Autodesk Inventor part; units mm, degrees
ref_plane "YZ Plane" through (0, 0, 0) normal (1, 0, 0) x (0, 1, 0)
ref_plane "XZ Plane" through (0, 0, 0) normal (0, 1, 0) x (-1, 0, 0)
ref_plane "XY Plane" through (0, 0, 0) normal (0, 0, 1) x (1, 0, 0)
sketch "Sketch1" plane through (0, 0, 0) normal (0, 0, 1) x (1, 0, 0)
  line L0 (-107.95, 44.45) -> (107.95, 44.45)
  line L1 (-107.95, -54.45) -> (-72.95, -54.45)
  line L2 (-72.95, -54.45) -> (-67.95, -44.45)
  line L3 (67.95, -44.45) -> (-67.95, -44.45)
  line L4 (107.95, -54.45) -> (72.95, -54.45)
  line L5 (72.95, -54.45) -> (67.95, -44.45)
  line L6 (-107.95, 44.45) -> (-107.95, -54.45)
  line L7 (107.95, 44.45) -> (107.95, -54.45)
  point P0 (0, 0)
  dimension "d36" = 88.9
  dimension "d38" = 215.9
  dimension "d39" = 44.45
  dimension "d40" = 107.95
  dimension "d41" = 98.9
  dimension "d42" = 10
  dimension "d43" = 116.565
  dimension "d44" = 35
  dimension "d45" = 35
  dimension "d46" = 116.565
  dimension "d47" = 40
extrude "Face ext" add sketch "Sketch1" along normal blind 3
sketch "Cutouts - skt" plane through (0, 0, 3) normal (0, 0, 1) x (1, 0, 0)
  line L0 (107.95, 44.45) -> (-107.95, 44.45)
  line L1 (63.8676, -13.289) -> (63.8676, -1.2663)
  line L2 (75.89, -13.289) -> (63.8676, -13.289)
  line L3 (75.89, -1.2663) -> (75.89, -13.289)
  line L4 (63.8676, -1.2663) -> (75.89, -1.2663)
  line L5 (46.0028, 16.7255) -> (58.0255, 16.7255)
  line L6 (46.0028, 4.7026) -> (46.0028, 16.7255)
  line L7 (58.0255, 4.7026) -> (46.0028, 4.7026)
  line L8 (58.0255, 16.7255) -> (58.0255, 4.7026)
  line L9 (75.9748, 33.8704) -> (75.9748, 21.8478)
  line L10 (63.9944, 33.8704) -> (75.9748, 33.8704)
  line L11 (63.9944, 21.8478) -> (63.9944, 33.8704)
  line L12 (75.9748, 21.8478) -> (63.9944, 21.8478)
  line L13 (63.9521, 16.7677) -> (75.9324, 16.7677)
  line L14 (63.9521, 4.7874) -> (63.9521, 16.7677)
  line L15 (75.9324, 4.7874) -> (63.9521, 4.7874)
  line L16 (75.9324, 16.7677) -> (75.9324, 4.7874)
  line L17 (94.0088, 4.8721) -> (94.0088, 16.8525)
  line L18 (82.0285, 4.8721) -> (94.0088, 4.8721)
  line L19 (82.0285, 16.8525) -> (82.0285, 4.8721)
  line L20 (94.0088, 16.8525) -> (82.0285, 16.8525)
  line L21 (27.7989, -11.6866) -> (-67.95, -11.6866)
  line L22 (-67.95, 28.3134) -> (25.7989, 28.3134)
  line L23 (32.0499, 28.3134) -> (32.0499, -11.6866)
  circle A0 centre (-85.95, 18.45) radius 8
  circle A1 centre (-85.95, -21.55) radius 8
  line L24 (-67.95, 28.3134) -> (32.0499, 28.3134)
  line L25 (32.0499, 28.3134) -> (32.0499, -11.6866)
  line L26 (32.0499, -11.6866) -> (-67.95, -11.6866)
  line L27 (-67.95, -11.6866) -> (-67.95, 28.3134)
  line L28 (63.9944, 33.8704) -> (75.9748, 33.8704)
  line L29 (75.9748, 33.8704) -> (75.9748, 21.8478)
  line L30 (75.9748, 21.8478) -> (63.9944, 21.8478)
  line L31 (63.9944, 21.8478) -> (63.9944, 33.8704)
  line L32 (82.0285, 16.8525) -> (94.0088, 16.8525)
  line L33 (94.0088, 16.8525) -> (94.0088, 4.8721)
  line L34 (94.0088, 4.8721) -> (82.0285, 4.8721)
  line L35 (82.0285, 4.8721) -> (82.0285, 16.8525)
  line L36 (63.9521, 16.7677) -> (75.9324, 16.7677)
  line L37 (75.9324, 16.7677) -> (75.9324, 4.7874)
  line L38 (75.9324, 4.7874) -> (63.9521, 4.7874)
  line L39 (63.9521, 4.7874) -> (63.9521, 16.7677)
  line L40 (46.0028, 16.7255) -> (58.0255, 16.7255)
  line L41 (58.0255, 16.7255) -> (58.0255, 4.7026)
  line L42 (58.0255, 4.7026) -> (46.0028, 4.7026)
  line L43 (46.0028, 4.7026) -> (46.0028, 16.7255)
  line L44 (63.8676, -1.2663) -> (75.89, -1.2663)
  line L45 (75.89, -1.2663) -> (75.89, -13.289)
  line L46 (75.89, -13.289) -> (63.8676, -13.289)
  line L47 (63.8676, -13.289) -> (63.8676, -1.2663)
  line L48 (-36.7815, -30.9654) -> (-26.011, -30.9654)
  line L49 (-26.011, -30.9654) -> (-26.011, -40.9281)
  line L50 (-26.011, -40.9281) -> (-36.7815, -40.9281)
  line L51 (-36.7815, -40.9281) -> (-36.7815, -30.9654)
  line L52 (-16.5867, -34.4658) -> (45.1738, -34.4658) construction
  line L53 (45.1738, -34.4658) -> (45.1738, -38.1955) construction
  line L54 (45.1738, -38.1955) -> (-16.5867, -38.1955) construction
  line L55 (-16.5867, -38.1955) -> (-16.5867, -34.4658) construction
  line L56 (-107.95, 44.45) -> (-107.95, -54.45)
  point P0 (-107.95, -44.45)
  point P1 (0, 0)
  point P2 (-70.7327, 35.8725)
  point P3 (22.3305, 35.8725)
  point P4 (22.3305, -19.1888)
  point P5 (-70.7327, -19.1888)
  point P6 (48.035, 31.7962)
  point P7 (92.0616, 31.7962)
  point P8 (48.035, -12.2207)
  point P9 (92.0616, -12.2207)
  point P10 (48.035, 31.7962)
  point P11 (92.0616, 31.7962)
  point P12 (92.0616, -12.2207)
  point P13 (48.035, -12.2207)
  point P14 (-70.7327, 35.8725)
  point P15 (22.3305, 35.8725)
  point P16 (22.3305, -19.1888)
  point P17 (-70.7327, -19.1888)
  dimension "d8" = 16
  dimension "d9" = 16
  dimension "d13" = 26
  dimension "d48" = 40
  dimension "d49" = 99.9999
  dimension "d50" = 40
  dimension "d51" = 93.0632
  dimension "d52" = 93.0632
  dimension "d53" = 55.0612
  dimension "d54" = 55.0612
  dimension "d55" = 8.5775
  dimension "d57" = 7.5591
  dimension "d59" = 44.0266
  dimension "d60" = 44.0266
  dimension "d61" = 22
  dimension "d62" = 22
  dimension "d90" = 40
  dimension "d91" = 18
sketch3d "3D Sketch1"
extrude "Cut-outs ext" cut sketch "Cutouts - skt" against normal through all
hole "Hole1" at (-70.7327, 35.8725, 3) at (-70.7327, -19.1888, 3) at (22.3305, -19.1888, 3) at (22.3305, 35.8725, 3) at (48.035, -12.2207, 3) at (48.035, 31.7962, 3) at (92.0616, 31.7962, 3) at (92.0616, -12.2207, 3) direction (0, 0, -1) diameter 3 end through all
sketch "Mating Holes" plane through (0, 0, 3) normal (0, 0, 1) x (1, 0, 0)
  line L0 (107.95, 44.45) -> (-107.95, 44.45)
  line L1 (-107.95, 44.45) -> (-107.95, -54.45)
  line L2 (-67.95, -44.45) -> (67.95, -44.45)
  line L3 (107.95, -54.45) -> (107.95, 44.45)
  circle A0 centre (-103.95, 0) radius 1.5
  line L4 (-105.5, -6) -> (-102.4, -6)
  line L5 (-102.4, -6) -> (-102.4, -16.1)
  line L6 (-102.4, -16.1) -> (-105.5, -16.1)
  line L7 (-105.5, -16.1) -> (-105.5, -6)
  line L8 (-105.5, 16.0999) -> (-102.4, 16.0999)
  line L9 (-102.4, 16.0999) -> (-102.4, 5.9999)
  line L10 (-102.4, 5.9999) -> (-105.5, 5.9999)
  line L11 (-105.5, 5.9999) -> (-105.5, 16.0999)
  circle A1 centre (103.95, 0) radius 1.5
  line L12 (102.4, -6) -> (105.5, -6)
  line L13 (105.5, -6) -> (105.5, -16.1)
  line L14 (105.5, -16.1) -> (102.4, -16.1)
  line L15 (102.4, -16.1) -> (102.4, -6)
  line L16 (102.4, 16.0999) -> (105.5, 16.0999)
  line L17 (105.5, 16.0999) -> (105.5, 5.9999)
  line L18 (105.5, 5.9999) -> (102.4, 5.9999)
  line L19 (102.4, 5.9999) -> (102.4, 16.0999)
  point P0 (0, 0)
  dimension "d63" = 3
  dimension "d75" = 44.45
  dimension "d79" = 3.1
  dimension "d80" = 10.1
  dimension "d81" = 6
  dimension "d85" = 3.1
  dimension "d86" = 10.1
  dimension "d87" = 5.9999
  dimension "d88" = 1.55
  dimension "d89" = 1.55
  dimension "d92" = 3
  dimension "d93" = 3.1
  dimension "d94" = 10.1
  dimension "d95" = 6
  dimension "d96" = 3.1
  dimension "d97" = 10.1
  dimension "d98" = 5.9999
  dimension "d99" = 1.55
  dimension "d100" = 1.55
  dimension "d101" = 4
  dimension "d102" = 44.45
  dimension "d103" = 4
  dimension "d104" = 88.9
extrude "Side Panel Slots" cut sketch "Mating Holes" against normal through all
sketch "Bottom Panel Slots" plane through (0, 0, 3) normal (0, 0, 1) x (1, 0, 0)
  line L0 (-107.95, 44.45) -> (-107.95, -54.45)
  line L1 (-107.95, -54.45) -> (-72.95, -54.45)
  line L2 (72.95, -54.45) -> (107.95, -54.45)
  circle A0 centre (-87.945, -41.45) radius 1.5
  line L3 (-93.945, -39.9) -> (-104.045, -39.9)
  line L4 (-104.045, -39.9) -> (-104.045, -43)
  line L5 (-104.045, -43) -> (-93.945, -43)
  line L6 (-93.945, -43) -> (-93.945, -39.9)
  line L7 (-81.945, -39.9) -> (-71.845, -39.9)
  line L8 (-71.845, -39.9) -> (-71.845, -43)
  line L9 (-71.845, -43) -> (-81.945, -43)
  line L10 (-81.945, -43) -> (-81.945, -39.9)
  circle A1 centre (87.013, -41.45) radius 1.5
  line L11 (93.013, -42.95) -> (103.113, -42.95)
  line L12 (103.113, -42.95) -> (103.113, -39.85)
  line L13 (103.113, -39.85) -> (93.013, -39.85)
  line L14 (93.013, -39.85) -> (93.013, -42.95)
  line L15 (81.013, -39.85) -> (70.913, -39.85)
  line L16 (70.913, -39.85) -> (70.913, -42.95)
  line L17 (70.913, -42.95) -> (81.013, -42.95)
  line L18 (81.013, -42.95) -> (81.013, -39.85)
  circle A2 centre (-0.45, -41.45) radius 1.5
  line L19 (5.55, -42.95) -> (15.65, -42.95)
  line L20 (15.65, -42.95) -> (15.65, -39.85)
  line L21 (15.65, -39.85) -> (5.55, -39.85)
  line L22 (5.55, -39.85) -> (5.55, -42.95)
  line L23 (-6.45, -39.85) -> (-16.55, -39.85)
  line L24 (-16.55, -39.85) -> (-16.55, -42.95)
  line L25 (-16.55, -42.95) -> (-6.45, -42.95)
  line L26 (-6.45, -42.95) -> (-6.45, -39.85)
  point P0 (0, 0)
  point P1 (-93.945, -41.45)
  point P2 (-71.845, -41.45)
  dimension "d109" = 3
  dimension "d112" = 10.1
  dimension "d113" = 3.1
  dimension "d116" = 13
  dimension "d118" = 10.1
  dimension "d119" = 3.1
  dimension "d120" = 13
  dimension "d123" = 6
  dimension "d124" = 6
  dimension "d125" = 13
  dimension "d129" = 3
  dimension "d130" = 10.1
  dimension "d131" = 3.1
  dimension "d132" = 10.1
  dimension "d133" = 3.1
  dimension "d134" = 6
  dimension "d137" = 6
  dimension "d138" = 13
  dimension "d140" = 1.5
  dimension "d141" = 1.5
  dimension "d142" = 3
  dimension "d143" = 107.5
  dimension "d144" = 13
  dimension "d145" = 10.1
  dimension "d146" = 3.1
  dimension "d147" = 10.1
  dimension "d148" = 3.1
  dimension "d149" = 1.5
  dimension "d150" = 1.5
  dimension "d151" = 6
  dimension "d152" = 6
  dimension "d155" = 87.463
  dimension "d156" = 87.495
extrude "Extrusion4" cut sketch "Bottom Panel Slots" against normal blind 10
equation "\"d45\" = d44"
equation "\"d46\" = d43"
equation "\"d62\" = d61"
equation "\"d75\" = 0.5 * d104"
equation "\"d79\" = d85"
equation "\"d80\" = d86"
equation "\"d88\" = 0.5 * d85"
equation "\"d89\" = d88"
equation "\"d93\" = d96"
equation "\"d94\" = d97"
equation "\"d99\" = 0.5 * d96"
equation "\"d100\" = d99"
equation "\"d101\" = d84"
equation "\"d102\" = d75"
equation "\"d105\" = d76"
properties part number "Front Panel"
Verification items for the finished model (mm, model axes). A direction names the side the tool comes from. Give positions to 0.01 mm unless a question says otherwise; leave off trailing zeros. Order: outer loops, then holes, each group sorted by start corner. A loop starts at its lowest first (then second) coordinate and runs counter-clockwise, first axis right, second up. Notation, with made-up numbers: (-16.5, -13.75) -> (42.5, -13.75) arc R22 cw to (42.5, -0.75) -> close; hole circle Ø1 at (73.5, -5.5). An arc over 180 degrees is marked (long way). One line per item, written item: value.
(1) Sectioned sample at A-A on y = -33. Record the cut outline in (x, z), then the cut area to 3 significant figures.
Final values:
outline: (-107.95, 0) -> (-36.78, 0) -> (-36.78, 3) -> (-107.95, 3) -> close; (-26.01, 0) -> (107.95, 0) -> (107.95, 3) -> (-26.01, 3) -> close
area: 615 mm^2
(2) Draft check along X on faces 1 (the face through (-2, -15, 0)), 2 (the face through (70.485, -49.52, 1.479)). Enter one of: pulls with the +X half, pulls with the -X half, needs draft (parallel to the pull), parting line crosses it, or undercut.
Final values:
face 1: needs draft
face 2: undercut
(3) Tool access check on faces 3 (the face through (-78.56, -24.61, 1.52)), 4 (the face through (-70.485, -49.52, 1.479)). Record the directions out of +Z, -Z, +X, -X, +Y, -Y that give a thin tool (end or side, any length) a straight path to the whole face; none if there is none.
Final values:
face 3: +Z, -Z
face 4: +Z, -Z, -Y
(4) Scan lines: line 1 along Y through (x, z) = (87, 2.65); line 2 along Y through (x, z) = (9.5, 0.7); line 3 along X through (y, z) = (-7.5, 2.3). Record each from-to range of solid material in increasing order. Write a range as [from, to].
Final values:
line 1: [-54.45, -42.95], [-39.95, 4.87], [16.85, 44.45]
line 2: [-44.45, -42.95], [-39.85, -11.69], [28.31, 44.45]
line 3: [-107.95, -105.5], [-102.4, -67.95], [32.05, 63.87], [75.89, 102.4], [105.5, 107.95]
(5) Sectioned sample at D-D on x = -29. Record the cut outline in (y, z).
Final values:
outline: (-44.45, 0) -> (-40.93, 0) -> (-40.93, 3) -> (-44.45, 3) -> close; (-30.97, 0) -> (-11.69, 0) -> (-11.69, 3) -> (-30.97, 3) -> close; (28.31, 0) -> (44.45, 0) -> (44.45, 3) -> (28.31, 3) -> close
(6) Gauge pin test, flat end, axial feed: pin 1 (0.9 mm diameter, centred on x = -30.5, z = 2, fed in from -Y). Record the tip position at first contact, or that the pin passes through.
Final values:
pin 1: y = -44.45
(7) Sectioned sample at C-C on y = 8.5. Record the cut outline in (x, z).
Final values:
outline: (-107.95, 0) -> (-105.5, 0) -> (-105.5, 3) -> (-107.95, 3) -> close; (-102.4, 0) -> (-67.95, 0) -> (-67.95, 3) -> (-102.4, 3) -> close; (32.05, 0) -> (46, 0) -> (46, 3) -> (32.05, 3) -> close; (58.03, 0) -> (63.95, 0) -> (63.95, 3) -> (58.03, 3) -> close; (75.93, 0) -> (82.03, 0) -> (82.03, 3) -> (75.93, 3) -> close; (94.01, 0) -> (102.4, 0) -> (102.4, 3) -> (94.01, 3) -> close; (105.5, 0) -> (107.95, 0) -> (107.95, 3) -> (105.5, 3) -> close
(8) Sectioned sample at B-B on x = 53.5. Record the cut outline in (y, z).
Final values:
outline: (-44.45, 0) -> (4.7, 0) -> (4.7, 3) -> (-44.45, 3) -> close; (16.73, 0) -> (44.45, 0) -> (44.45, 3) -> (16.73, 3) -> close
